from build123d import *

# Parameters (mm, degrees)
SKETCH1_W           = 126.042151156
SKETCH1_H           = 152.641955782
BOSS_EXTRUDE1_DEPTH = 24
SKETCH2_W           = 126.042151156
SKETCH2_H           = 17.009297173
BOSS_EXTRUDE2_DEPTH = 62
RIB1_REACH          = 172.609
SKETCH3_WALL_W      = 492.350042414
SKETCH3_WALL_H      = 100


with BuildPart() as part:
    # Sketch1 → Boss-Extrude1 (new body)
    with BuildSketch(Plane(origin=(0, 0, 0), x_dir=(1, 0, 0), z_dir=(0, 1, 0))):
        Rectangle(SKETCH1_W, SKETCH1_H)
    extrude(amount=BOSS_EXTRUDE1_DEPTH)

    # Sketch2 → Boss-Extrude2 (add)
    with BuildSketch(Plane(origin=(0, 24, 0), x_dir=(1, 0, 0), z_dir=(0, 1, 0))):
        with Locations((0, 67.816329305)):
            Rectangle(SKETCH2_W, SKETCH2_H)
    extrude(amount=BOSS_EXTRUDE2_DEPTH)

    # Sketch3 wall → Rib1 (add, up to next)
    with BuildSketch(Plane(origin=(63.021075578, 55, 8.504648587), x_dir=(0, -0.415740341777, 0.909483352359), z_dir=(0, -0.909483352359, -0.415740341777)), mode=Mode.PRIVATE) as rib1_sk1:
        with Locations((0, 50)):
            Rectangle(SKETCH3_WALL_W, SKETCH3_WALL_H)
    rib1_tool1 = extrude(rib1_sk1.sketch, amount=RIB1_REACH, mode=Mode.PRIVATE) - part.part
    add(rib1_tool1.solids().sort_by_distance((63.021075578, 55, 8.504648587))[0])


solid = part.part
Geometry: final body of the model. Coordinates: model frame, mm. A direction names the side the tool comes from. Give positions to 0.01 mm unless a question says otherwise; leave off trailing zeros. Write each loop counter-clockwise with the first axis right and the second up, starting at its lowest first coordinate (ties: lowest second). Pieces come first, ordered by that corner, then holes. Notation, with made-up numbers: (-39, 70) - (-15, 70) arc R36 ccw to (-15, 104) - close; hole circle Ø3 at (24, -15.75). An arc over 180 degrees is marked (long way). Return JSON: item names as keys, results as strings. Group by question number.
1) Section B-B on z = 43.5. Return the cut outline in (x, y).
2) Set-up query: faces 1 (the flat face through (-1, 86, -68)), 2 (the flat face through (-50, 55, -59.312)). Return all of +Z, -Z, +X, -X, +Y, -Y with unobstructed straight access to the full face (end or side cutting, diameter ignored); none if empty.
3) Line query: line 1 (Y direction, x = -42.5, z = 6); line 2 (Z direction, x = -44, y = 39.5); line 3 (X direction, y = 53.5, z = -18.5). Output: solid intervals per line, ascending.
4) First-contact query: P1, Ø2, axis at x = 10, y = 56.5, coming from the +Z side; P2, Ø3, axis at y = 56, z = -17, coming from the -X side; P3, Ø12, axis at x = 33, y = 46.5, coming from the +Z side. Flat tips, straight axial feed; report the tip coordinate or a pass-through.
5) Section C-C on y = 52. Return the cut outline in (x, z), plus the area to 3 significant figures.
6) Section A-A on x = 25.5. Return the cut outline in (y, z).
Filled in:
{
 "1": {"outline": "(-63.02, 0) - (63.02, 0) - (63.02, 39) - (-36.98, 39) - (-36.98, 24) - (-63.02, 24) - close"},
 "2": {"face 1": "+Z, -Z, +X, -X, +Y", "face 2": "+Z, -X, +Y"},
 "3": {"line 1": "y = 0 to 24", "line 2": "z = -76.32 to -59.31", "line 3": "x = -36.98 to 63.02"},
 "4": {"P1": "stops at z = 7.41", "P2": "stops at x = -36.98", "P3": "stops at z = 40.23"},
 "5": {"outline": "(-63.02, -76.32) - (63.02, -76.32) - (63.02, 15.07) - (-36.98, 15.07) - (-36.98, -59.31) - (-63.02, -59.31) - close", "area": "9,580 mm^2"},
 "6": {"outline": "(0, -76.32) - (86, -76.32) - (86, -59.31) - (24, 76.32) - (0, 76.32) - close"}
}
